from build123d import *

# Parameters (mm, degrees)
SKETCH1_R           = 2.5
REVOLVE1_ANGLE      = 180
SKETCH1_2_R         = 2.5
BOSS_EXTRUDE1_DEPTH = 80
SKETCH2_R           = 2.5
BOSS_EXTRUDE2_DEPTH = 80
CHAMFER1_SIZE       = 0.5


with BuildPart() as part:
    # Sketch1 → Revolve1 (revolve)
    with BuildSketch(Plane.XY):
        with Locations((0, 32)):
            Circle(SKETCH1_R)
    revolve(axis=Axis((0, 0, 0), (1, 0, 0)), revolution_arc=REVOLVE1_ANGLE)

    # Sketch1_2 → Boss-Extrude1 (add)
    with BuildSketch(Plane.XY):
        with Locations((0, 32)):
            Circle(SKETCH1_2_R)
    extrude(amount=-BOSS_EXTRUDE1_DEPTH)

    # Sketch2 → Boss-Extrude2 (add)
    with BuildSketch(Plane(origin=(0, 0, 0), x_dir=(-1, 0, 0), z_dir=(0, 0, -1))):
        with Locations(Location((0, -32, 0), (0, 0, 270))):
            Circle(SKETCH2_R)
    extrude(amount=BOSS_EXTRUDE2_DEPTH)

    # Chamfer1
    chamfer1_edges = [part.edges().sort_by_distance(p)[0] for p in [
        (0, -29.5, -80),
        (-2.5, 32, -80),
    ]]
    chamfer(chamfer1_edges, length=CHAMFER1_SIZE)


solid = part.part
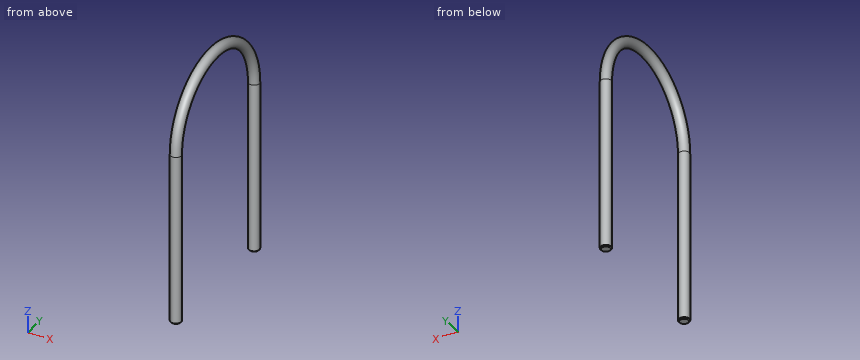
Design review of the part built by this model. Coordinates are the model's own, in mm. Coordinates: 2 decimals unless noted, no trailing zeros. Loops run counter-clockwise (first coordinate to the right, second up) from the corner with the lowest first, then second, coordinate; pieces in that order, holes last. Notation, with made-up numbers: (-34, -32.5) -> (14, -32.5) arc R16 ccw to (14, -28.5) -> close; hole circle Ø9 at (-40, 31). An arc over 180 degrees is marked (long way). Use a Markdown table: item, result. Add a question column.
Item 1: We need section B-B, the plane x = 0. Write out the cut boundary in (y, z), and give its area (3 significant figures).
Item 2: Clearance check with flat-ended pins moving along their axes: P1, Ø1.5, axis at x = 1, z = 9.5, coming from the -Y side; P2, Ø3, axis at x = -1.5, z = -64, coming from the +Y side; P3, Ø2, axis at x = 1, z = 12, coming from the +Y side. State where each tip first meets the part, or that it passes through.
Item 3: Wall thickness on L1, parallel to Y at x = 1.2, z = 9.5; L2, parallel to Y at x = -0.8, z = 27; L3, parallel to X at y = 30, z = 5.5: over which ranges is each line inside the solid? List them lowest first. Write a range as from..to.
Item 4: We need section A-A, the plane z = -46.5. Write out the cut boundary in (x, y).
Numbers:
| question | item | result |
|---|---|---|
| 1 | outline | (-34.5, -79.5) -> (-34, -80) -> (-30, -80) -> (-29.5, -79.5) -> (-29.5, 0) arc R29.5 cw to (29.5, 0) -> (29.5, -79.5) -> (30, -80) -> (34, -80) -> (34.5, -79.5) -> (34.5, 0) arc R34.5 ccw to (-34.5, 0) -> close |
| 1 | area | 1,300 mm^2 |
| 2 | P1 | stops at y = -33.27 |
| 2 | P2 | stops at y = 34.5 |
| 2 | P3 | stops at y = 32.6 |
| 3 | L1 | y = -32.85..-28.25, 28.25..32.85 |
| 3 | L2 | y = -21.26..-12.21, 12.21..21.26 |
| 3 | L3 | x = -2..2 |
| 4 | outline | circle Ø5 at (0, -32); circle Ø5 at (0, 32) |
